Autodesk Inventor part; units mm, degrees
ref_plane "YZ Plane" through (0, 0, 0) normal (1, 0, 0) x (0, 1, 0)
ref_plane "XZ Plane" through (0, 0, 0) normal (0, 1, 0) x (-1, 0, 0)
ref_plane "XY Plane" through (0, 0, 0) normal (0, 0, 1) x (1, 0, 0)
sketch "TopProfile" plane through (0, 0, 0) normal (0, 0, 1) x (1, 0, 0)
  circle A0 centre (0, 0) radius 3
  circle A1 centre (0, 0) radius 5 construction
  line L0 (-2, -4.4651) -> (-2, -15.4651)
  line L1 (-2, -15.4651) -> (2, -15.4651)
  line L2 (2, -15.4651) -> (2, -4.4651)
  line L3 (-2, -4.4651) -> (2, -4.4651)
  line L4 (2.25, -4.4651) -> (-2.25, -4.4651) construction
  line L5 (5, -4.4651) -> (-5, -4.4651)
  line L6 (5, 0) -> (5, -4.4651)
  line L7 (-5, 0) -> (-5, -4.4651)
  arc A2 (5, 0) -> (-5, 0) centre (0, 0) ccw
  dimension "d0" = 6
  dimension "d1" = 10
  dimension "d3" = 4
  dimension "d5" = 11
  dimension "d8" = 4.5
  dimension "d9" = 0.25
extrude "TopProfileFeature" add sketch "TopProfile" along normal blind 9
chamfer "BodyChamferFeatures" distance 2 angle 45 2 edges at (0, -15.4651, 9) (0, -15.4651, 0)
sketch "MountRail" plane through (2, -13.4651, 9) normal (1, 0, 0) x (0, 0, -1)
  line L0 (0, 0) -> (0, 9) construction
  line L1 (0, 2) -> (9, 2) construction
  arc A0 (5, 0) -> (5, 4) centre (5, 2) ccw
  arc A1 (4, 4) -> (4, 0) centre (4, 2) ccw
  line L2 (5, 4) -> (4, 4)
  line L3 (5, 0) -> (4, 0)
  line L4 (7, -2) -> (2, -2) construction
  line L5 (9, 9) -> (9, 0) construction
  point P0 (9, -2)
  dimension "d41" = 2
  dimension "d43" = 4
  dimension "d44" = 4
  dimension "d55" = 4
extrude "MountRailFeature" cut sketch "MountRail" against normal through all
properties part number "ForearmCuffConnector"
Build history of the part. All positions in model axes, mm. A direction names the side the tool comes from. Round coordinates to 2 decimals unless told otherwise and drop trailing zeros. Loops run counter-clockwise (first coordinate to the right, second up) from the corner with the lowest first, then second, coordinate; pieces in that order, holes last.
Item 1: Saw through at B-B (z = 4.25). List the corners of the cut face in (x, y).
Item 2: Saw through at A-A (x = 0). List the corners of the cut face in (y, z), then the cut area to 3 significant figures.
Item 3: Saw through at D-D (x = 1). List the corners of the cut face in (y, z), then the cut area to 3 significant figures.
Item 4: Pin check, flat tips, straight feed: P1, Ø5, axis at x = 0, y = 0, coming from the +Z side; P2, Ø1.5, axis at y = -9, z = 2.5, coming from the -X side; P3, Ø4.5, axis at y = -8, z = 6, coming from the +X side; P4, Ø1.5, axis at x = 3, z = 4, coming from the -Y side. Stop position of each tip, or through.
Item 5: Saw through at C-C (y = -11.75). List the corners of the cut face in (x, z).
Item 6: Two-plate mould, pull along Y, no slides. Class faces 1 (the face through (0, -4, 0)), 2 (the face through (0, -9.465, 4.5)), 3 (the face through (0.028, -14.451, 8.014)): released by +Y, released by -Y, zero draft, split by the parting line, or undercut.
Item 7: Drill centre lines: line 1 along Y through (x, z) = (0, 4.25); line 2 along Y through (x, z) = (0, 3.5); line 3 along X through (y, z) = (-13.5, 8). Where is each one in solid material? Low to high.
Item 8: Which spindle directions (+Z, -Z, +X, -X, +Y, -Y) get a long thin tool onto all of the face, cutting with end or side? Do faces 4 (the face through (4, -4.465, 4)), 5 (the face through (-2, -9, 4)), 6 (the face through (0, -11.4, 7)). Say none if no direction does.
Worked answers:
1. outline: (-5, -4.47) - (-2, -4.47) - (-2, -9.47) - (2, -9.47) - (2, -4.47) - (5, -4.47) - (5, 0) arc R5 ccw to (-5, 0) - close; (-2, -15.47) - (2, -15.47) - (2, -13.47) - (-2, -13.47) - close; hole circle Ø6 at (0, 0)
2. outline: (-15.47, 2) - (-13.47, 0) - (-3, 0) - (-3, 9) - (-13.47, 9) - (-15.47, 7) - close; (3, 0) - (5, 0) - (5, 9) - (3, 9) - close; hole (-13.47, 4) arc R2 ccw to (-9.47, 4) - (-9.47, 5) arc R2 ccw to (-13.47, 5) - close
2. area: 110 mm2
3. outline: (-15.47, 2) - (-13.47, 0) - (-2.83, 0) - (-2.83, 9) - (-13.47, 9) - (-15.47, 7) - close; (2.83, 0) - (4.9, 0) - (4.9, 9) - (2.83, 9) - close; hole (-13.47, 4) arc R2 ccw to (-9.47, 4) - (-9.47, 5) arc R2 ccw to (-13.47, 5) - close
3. area: 112 mm2
4. P1: passes through
4. P2: stops at x = -2
4. P3: stops at x = 2
4. P4: stops at y = -4.47
5. outline: (-2, 0) - (2, 0) - (2, 2.02) - (-2, 2.02) - close; (-2, 6.98) - (2, 6.98) - (2, 9) - (-2, 9) - close
6. face 1: zero draft
6. face 2: undercut
6. face 3: released by -Y
7. line 1: y = -15.47 to -13.47, -9.47 to -3, 3 to 5
7. line 2: y = -15.47 to -13.4, -9.53 to -3, 3 to 5
7. line 3: x = -2 to 2
8. face 4: +Z, -Z, +X, -Y
8. face 5: +Z, -Z, -X, -Y
8. face 6: +X, -X
